Can you work these out from the model? Positions are in its coordinate system, mm. A direction names the side the tool comes from. Coordinates: 2 decimals unless noted, no trailing zeros. Answer as CSV lines item,"result". Start each with the question number.
1. If we mould it in two halves opening along Y, with no side actions, what happens to faces 4 (the face through (0, 40, -17.467)), 5 (the face through (1.74, 38.16, 16.99)), 6 (the face through (0, 42, 32.5))? For each: released by +Y, released by -Y, zero draft, split by the parting line, or undercut.
2. I need wall thicknesses on line 1 along Y through (x, z) = (0, -28); line 2 along Y through (x, z) = (-18, 4); line 3 along X through (y, z) = (39.75, 17). Which ranges of each line are inside material? Lowest first, please. Write a range as from..to.
3. Will these pins go through, and if not, where does the flat tip stop? pin 1 (1 mm diameter, centred on x = -0.5, z = 13.5, fed in from -Y); pin 2 (1.3 mm diameter, centred on x = 0, y = 40, fed in from +Z); pin 3 (0.8 mm diameter, centred on x = 1, y = 39, fed in from -Z).
4. On a 3-axis mill with a long thin cutter (end or side, diameter ignored), from which of +Z, -Z, +X, -X, +Y, -Y can I reach the whole of each face in a straight line? I mean faces 1 (the face through (1.74, 38.16, -16.99)), 2 (the face through (0, 40, 17.467)), 3 (the face through (-0.028, 38.239, 15.998)). Say none if no direction works.
```python
from build123d import *

# Parameters (mm, degrees)
SKETCH1_W               = 60
SKETCH1_H               = 65
SKETCH1_W_2             = 55
SKETCH1_H_2             = 60
BOSS_EXTRUDE1_DEPTH     = 40
SKETCH2_W               = 60
SKETCH2_H               = 65
BOSS_EXTRUDE2_DEPTH     = 2.5
BOSS_EXTRUDE3_DEPTH     = 65
CUT_EXTRUDE1_REACH      = 83.03
CUT_EXTRUDE2_DEPTH      = 84.873058845
CUT_EXTRUDE2_DEPTH_BACK = 84.873058845
SKETCH5_W               = 60
SKETCH5_H               = 41
SNAP_START              = -17.466738465
SNAP_HOOK1_DEPTH        = 0.923076923
SNAP_START_2            = -1.762465991
SNAP_HOOK1_2_DEPTH      = 3.524931982
SNAP_START_3            = -1.989936516
SNAP_HOOK1_3_DEPTH      = 3.979873032
SNAP_START_4            = -19
SNAP_HOOK1_4_DEPTH      = 5


with BuildPart() as part:
    # Sketch1 → Boss-Extrude1 (new body)
    with BuildSketch(Plane(origin=(0, 0, 0), x_dir=(1, 0, 0), z_dir=(0, 1, 0))):
        Rectangle(SKETCH1_W, SKETCH1_H)
        Rectangle(SKETCH1_W_2, SKETCH1_H_2, mode=Mode.SUBTRACT)
    extrude(amount=BOSS_EXTRUDE1_DEPTH)

    # Sketch2 → Boss-Extrude2 (add)
    with BuildSketch(Plane(origin=(0, 40, 0), x_dir=(1, 0, 0), z_dir=(0, 1, 0))):
        Rectangle(SKETCH2_W, SKETCH2_H)
    extrude(amount=BOSS_EXTRUDE2_DEPTH)

    # Sketch3 → Boss-Extrude3 (add)
    with BuildSketch(Plane(origin=(0, 0, -32.5), x_dir=(-1, 0, 0), z_dir=(0, 0, -1))):
        Polygon((-30, 42.5), (-28.8, 43.7), (-27.6, 42.5), (-26.4, 43.7), (-25.2, 42.5), (-24, 43.7), (-22.8, 42.5), (-21.6, 43.7), (-20.4, 42.5), (-19.2, 43.7), (-18, 42.5), (-16.8, 43.7), (-15.6, 42.5), (-14.4, 43.7), (-13.2, 42.5), (-12, 43.7), (-10.8, 42.5), (-9.6, 43.7), (-8.4, 42.5), (-7.2, 43.7), (-6, 42.5), (-4.8, 43.7), (-3.6, 42.5), (-2.4, 43.7), (-1.2, 42.5), (0, 43.7), (1.2, 42.5), (2.4, 43.7), (3.6, 42.5), (4.8, 43.7), (6, 42.5), (7.2, 43.7), (8.4, 42.5), (9.6, 43.7), (10.8, 42.5), (12, 43.7), (13.2, 42.5), (14.4, 43.7), (15.6, 42.5), (16.8, 43.7), (18, 42.5), (19.2, 43.7), (20.4, 42.5), (21.6, 43.7), (22.8, 42.5), (24, 43.7), (25.2, 42.5), (26.4, 43.7), (27.6, 42.5), (28.8, 43.7), (30, 42.5), (30, 42.170064374), (-30, 42.170064374), align=None)
    extrude(amount=-BOSS_EXTRUDE3_DEPTH)

    # Cut-Extrude1: up to this face of the body (flat: up to its plane)
    cut_extrude1_end = Plane(part.part.faces().sort_by_distance((30, 21.25, 0))[0])
    # Sketch4 → Cut-Extrude1 (cut, up to the picked face)
    with BuildSketch(Plane.ZY.offset(30), mode=Mode.PRIVATE) as cut_extrude1_sk1:
        with BuildLine():
            Line((-32.5, 42.5), (-32.5, 43.7))
            Line((-32.5, 43.7), (-31.3, 43.7))
            ThreePointArc((-31.3, 43.7), (-32.148528137, 43.348528137), (-32.5, 42.5))
        make_face()
    cut_extrude1_tool1 = split(extrude(cut_extrude1_sk1.sketch, amount=-CUT_EXTRUDE1_REACH, mode=Mode.PRIVATE), bisect_by=cut_extrude1_end, keep=Keep.BOTH, mode=Mode.PRIVATE)
    cut_extrude1 = cut_extrude1_tool1.solids().sort_by(Axis((-30, 43.431958, -32.231958), (1, 0, 0)))[0]
    add(cut_extrude1, mode=Mode.SUBTRACT)

    # Mirror1: Cut-Extrude1 across plane
    add(cut_extrude1.mirror(Plane.XY), mode=Mode.SUBTRACT)

    # Sketch5 → Cut-Extrude2 (cut, two sides: drawn at the far end of the back side and taken through both)
    with BuildSketch(Plane.XY.offset(32.5).offset(-CUT_EXTRUDE2_DEPTH_BACK)):
        with Locations((0, 20.5)):
            Rectangle(SKETCH5_W, SKETCH5_H)
    extrude(amount=CUT_EXTRUDE2_DEPTH + CUT_EXTRUDE2_DEPTH_BACK, mode=Mode.SUBTRACT)

    # Snap Hook1: read off the stored shape, not the designer's step
    # Snap Hook1 outline → Snap Hook1 (add)
    with BuildSketch(Plane.XY.offset(SNAP_START)):
        Polygon((-1.5, 35.4), (1.5, 35.4), (1.989936516, 41), (-1.989936516, 41), align=None)
    snap_hook1 = extrude(amount=SNAP_HOOK1_DEPTH)

    # Snap Hook1 2 outline → Snap Hook1 2 (add)
    with BuildSketch(Plane.YZ.offset(SNAP_START_2)):
        Polygon((38.4, -17.466738465), (35.4, -17.466738465), (37.9, -18.466738465), (38.4, -18.466738465), align=None)
        Polygon((35.4, -16.543661542), (41, -16.543661542), (41, -15.466738465), align=None)
    snap_hook1_2 = extrude(amount=SNAP_HOOK1_2_DEPTH)

    # Snap Hook1 3 outline → Snap Hook1 3 (add)
    with BuildSketch(Plane.YZ.offset(SNAP_START_3)):
        Polygon((35.4, -16.543661542), (41, -16.543661542), (41, -15.466738465), align=None)
    snap_hook1_3 = extrude(amount=SNAP_HOOK1_3_DEPTH)

    # Snap Hook1 4 outline → Snap Hook1 4 (cut)
    with BuildSketch(Plane.XY.offset(SNAP_START_4)):
        Polygon((-1.989936516, 41), (-1.989936516, 34), (-1.377515871, 34), align=None)
        Polygon((1.377515871, 34), (1.989936516, 34), (1.989936516, 41), align=None)
    snap_hook1_4 = extrude(amount=SNAP_HOOK1_4_DEPTH, mode=Mode.SUBTRACT)

    # Mirror2: Snap Hook1, Snap Hook1 2, Snap Hook1 3, Snap Hook1 4 across plane
    add(snap_hook1.mirror(Plane.XY))
    add(snap_hook1_2.mirror(Plane.XY))
    add(snap_hook1_3.mirror(Plane.XY))
    add(snap_hook1_4.mirror(Plane.XY), mode=Mode.SUBTRACT)


solid = part.part
```
Solved:
1,face 4,"undercut"
1,face 5,"released by -Y"
1,face 6,"zero draft"
2,line 1,"41..43.7"
2,line 2,"41..42.5"
2,line 3,"-1.88..1.88"
3,pin 1,"y = 41"
3,pin 2,"z = 17.47"
3,pin 3,"z = -17.47"
4,face 1,"+Z, -Z, +X, -Y"
4,face 2,"+Z, +X, -X"
4,face 3,"+X, -X, -Y"
